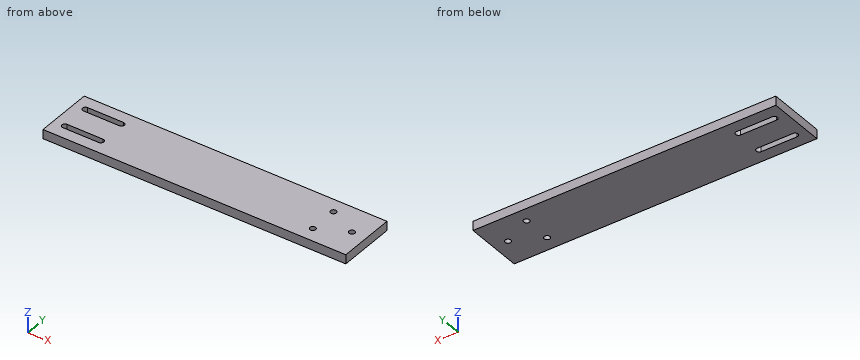
```python
from build123d import *

# Parameters (mm, degrees)
SKETCH1_W           = 210
SKETCH1_H           = 40
SKETCH1_R           = 2
BOSS_EXTRUDE1_DEPTH = 6.35


with BuildPart() as part:
    # Sketch1 → Boss-Extrude1 (new body)
    with BuildSketch(Plane.XY):
        with Locations((105, 20)):
            Rectangle(SKETCH1_W, SKETCH1_H)
        with Locations((180, 30)):
            Circle(SKETCH1_R, mode=Mode.SUBTRACT)
        with Locations((180, 10)):
            Circle(SKETCH1_R, mode=Mode.SUBTRACT)
        with Locations((200, 20)):
            Circle(SKETCH1_R, mode=Mode.SUBTRACT)
        with BuildLine():
            Line((8, 32), (33, 32))
            ThreePointArc((33, 32), (35, 30), (33, 28))
            Line((33, 28), (8, 28))
            ThreePointArc((8, 28), (6, 30), (8, 32))
        make_face(mode=Mode.SUBTRACT)
        with BuildLine():
            Line((8, 12), (33, 12))
            ThreePointArc((33, 12), (35, 10), (33, 8))
            Line((33, 8), (8, 8))
            ThreePointArc((8, 8), (6, 10), (8, 12))
        make_face(mode=Mode.SUBTRACT)
    extrude(amount=BOSS_EXTRUDE1_DEPTH)


solid = part.part
```
CAD build for the part. Positions are in the model's coordinates, mm. Give positions to 0.01 mm unless a question says otherwise; leave off trailing zeros. Loops run counter-clockwise (first coordinate to the right, second up) from the corner with the lowest first, then second, coordinate; pieces in that order, holes last. Notation, with made-up numbers: M 68.25,47 L 115.25,47 A18 cw 115.25,74 Z; hole C 6,-19 d5. An arc over 180 degrees is marked long. Use one line per item in the form item = value.
Item 1: Slice it at A-A (y = 30). List the corners of the cut face in (x, z), plus the area to 3 significant figures.
Determined:
outline = M 0,0 L 6,0 L 6,6.35 L 0,6.35 Z; M 35,0 L 178,0 L 178,6.35 L 35,6.35 Z; M 182,0 L 210,0 L 210,6.35 L 182,6.35 Z
area = 1,120 mm2
Item 2: Slice it at C-C (y = 20). List the corners of the cut face in (x, z), plus the area to 3 significant figures.
Determined:
outline = M 0,0 L 198,0 L 198,6.35 L 0,6.35 Z; M 202,0 L 210,0 L 210,6.35 L 202,6.35 Z
area = 1,310 mm2
Item 3: Slice it at D-D (z = 4). List the corners of the cut face in (x, y).
Determined:
outline = M 0,0 L 210,0 L 210,40 L 0,40 Z; hole M 8,8 L 33,8 A2 ccw 33,12 L 8,12 A2 ccw Z; hole M 8,28 L 33,28 A2 ccw 33,32 L 8,32 A2 ccw Z; hole C 180,10 d4; hole C 180,30 d4; hole C 200,20 d4
Item 4: Drill centre lines: probe 1 along Y at (x, z) = (180, 1.5); probe 2 along Y at (x, z) = (200, 2); probe 3 along X at (y, z) = (30.5, 5). Where is each one in solid material? Low to high. Write a range as from..to.
Determined:
probe_1 = 0..8, 12..28, 32..40
probe_2 = 0..18, 22..40
probe_3 = 0..6.06, 34.94..178.06, 181.94..210
Item 5: Slice it at B-B (x = 21). List the corners of the cut face in (y, z).
Determined:
outline = M 0,0 L 8,0 L 8,6.35 L 0,6.35 Z; M 12,0 L 28,0 L 28,6.35 L 12,6.35 Z; M 32,0 L 40,0 L 40,6.35 L 32,6.35 Z
